from build123d import *

# Parameters (mm, degrees)
SKETCH_1_R          = 50
EXTRUDE_1_DEPTH     = 8
SKETCH_2_W          = 10
SKETCH_2_H          = 10
CUT_EXTRUDE_1_DEPTH = 8
SKETCH_3_R          = 5
SKETCH_3_R_2        = 2
EXTRUDE_3_DEPTH     = 8


with BuildPart() as part:
    # 草图1 → 凸台-拉伸1 (new body)
    with BuildSketch(Plane.XY):
        Circle(SKETCH_1_R)
    extrude(amount=EXTRUDE_1_DEPTH)

    # 草图2 → 切除-拉伸1 (cut)
    with BuildSketch(Plane.XY.offset(8)):
        Rectangle(SKETCH_2_W, SKETCH_2_H)
    extrude(amount=-CUT_EXTRUDE_1_DEPTH, mode=Mode.SUBTRACT)

    # 草图3 → 凸台-拉伸3 (add)
    # profile 1 of 4: a face of its own
    with BuildSketch(Plane.XY.offset(8)):
        with Locations((0, 32)):
            Circle(SKETCH_3_R)
        with Locations((0, 32)):
            Circle(SKETCH_3_R_2, mode=Mode.SUBTRACT)
    # profile 2 of 4: a face of its own
    with BuildSketch(Plane.XY.offset(8)):
        with Locations((32, 0)):
            Circle(SKETCH_3_R)
        with Locations((32, 0)):
            Circle(SKETCH_3_R_2, mode=Mode.SUBTRACT)
    # profile 3 of 4: a face of its own
    with BuildSketch(Plane.XY.offset(8)):
        with Locations((0, -32)):
            Circle(SKETCH_3_R)
        with Locations((0, -32)):
            Circle(SKETCH_3_R_2, mode=Mode.SUBTRACT)
    # profile 4 of 4: a face of its own
    with BuildSketch(Plane.XY.offset(8)):
        with Locations((-32, 0)):
            Circle(SKETCH_3_R)
        with Locations((-32, 0)):
            Circle(SKETCH_3_R_2, mode=Mode.SUBTRACT)
    extrude(amount=EXTRUDE_3_DEPTH)


solid = part.part
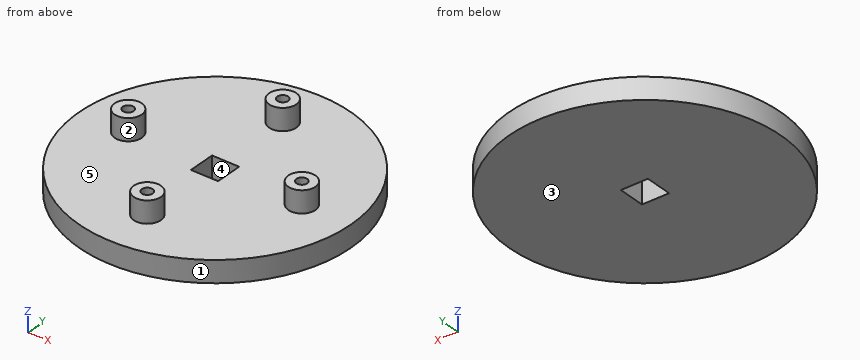
CAD build for the part. Positions are in the model's coordinates, mm. Face numbers are marked on the shaded views. A direction names the side the tool comes from. Coordinates: 2 decimals unless noted, no trailing zeros. Loops run counter-clockwise (first coordinate to the right, second up) from the corner with the lowest first, then second, coordinate; pieces in that order, holes last. Notation, with made-up numbers: (27, 60.5) - (77, 60.5) arc R10 ccw to (77, 69.5) - close; hole circle Ø5 at (4, 87.5). An arc over 180 degrees is marked (long way). Write item = value, one per line. Start each with the question number.
Q1. Drill centre lines: L1, parallel to Y at x = 0, z = 10; L2, parallel to Y at x = -32, z = 10.5; L3, parallel to Z at x = 22, y = -37.5. Where is each one in solid material? Low to high.
Q2. Cut at D-D, the plane x = -32. List the corners of the cut face in (y, z).
Q3. Pull direction X, two halves, no side cores. Call the marked faces 1, 2 and 3: pulls with the +X half, pulls with the -X half, needs draft (parallel to the pull), parting line crosses it, or undercut.
Q4. Cut at B-B, the plane y = 0. List the corners of the cut face in (x, z), then the cut area to 3 significant figures.
Q5. Cut at A-A, the plane z = 14.25. List the corners of the cut face in (x, y).
Q6. Which spindle directions (+Z, -Z, +X, -X, +Y, -Y) get a long thin tool onto all of the face, cutting with end or side? Do the marked faces 4 and 5. Say none if no direction does.
Q7. Flat gauge pins, fed straight in: pin 1 Ø3 at (x, z) = (-26.5, 3) entering from -Y; pin 2 Ø3 at (x, y) = (1, -31) entering from +Z; pin 3 Ø6 at (y, z) = (-38.5, 8) entering from -X; pin 4 Ø8 at (x, z) = (6.5, 13.5) entering from +Y. Where does each tip first touch, or does it go through?
Computed:
q1.L1 = -37 to -34, -30 to -27, 27 to 30, 34 to 37
q1.L2 = -5 to -2, 2 to 5
q1.L3 = 0 to 8
q2.outline = (-38.42, 0) - (38.42, 0) - (38.42, 8) - (5, 8) - (5, 16) - (2, 16) - (2, 8) - (-2, 8) - (-2, 16) - (-5, 16) - (-5, 8) - (-38.42, 8) - close
q3.face_1 = parting line crosses it
q3.face_2 = undercut
q3.face_3 = needs draft
q4.outline = (-50, 0) - (-5, 0) - (-5, 8) - (-27, 8) - (-27, 16) - (-30, 16) - (-30, 8) - (-34, 8) - (-34, 16) - (-37, 16) - (-37, 8) - (-50, 8) - close; (5, 0) - (50, 0) - (50, 8) - (37, 8) - (37, 16) - (34, 16) - (34, 8) - (30, 8) - (30, 16) - (27, 16) - (27, 8) - (5, 8) - close
q4.area = 816 mm²
q5.outline = circle Ø10 at (-32, 0); circle Ø10 at (0, -32); circle Ø10 at (0, 32); circle Ø10 at (32, 0); hole circle Ø4 at (-32, 0); hole circle Ø4 at (0, -32); hole circle Ø4 at (0, 32); hole circle Ø4 at (32, 0)
q6.face_4 = +Z, -Z
q6.face_5 = +Z
q7.pin_1 = -43.3
q7.pin_2 = 16
q7.pin_3 = -35.21
q7.pin_4 = 36.33
